```python
from build123d import *

# Parameters (mm, degrees)
CONG_1_R       = 1.1
ECHELLE1_SCALE = 0.69


with BuildPart() as part:
    # Esquisse1 → Révolution1 (revolve)
    with BuildSketch(Plane(origin=(0, 0, 0), x_dir=(0, 0, -1), z_dir=(1, 0, 0)), mode=Mode.PRIVATE) as r_volution1_sk:
        with BuildLine():
            Line((-7.5, 26), (-7.5, 21.2))
            Line((-7.5, 21.2), (-3.577708764, 21.2))
            ThreePointArc((-3.577708764, 21.2), (0, 22.8), (3.577708764, 21.2))
            Line((3.577708764, 21.2), (7.5, 21.2))
            Line((7.5, 21.2), (7.5, 26))
            Line((7.5, 26), (-7.5, 26))
        make_face()
    revolve(r_volution1_sk.sketch.rotate(Axis((0, 0, 0), (0, 0, -1)), 90), axis=Axis((0, 0, 0), (0, 0, -1)))

    # Congé1
    cong_1_edges = [part.edges().sort_by_distance(p)[0] for p in [
        (-26, 0, 7.5),
        (-26, 0, -7.5),
    ]]
    fillet(cong_1_edges, radius=CONG_1_R)


with BuildPart() as part_1:
    # Echelle1: scaled about (0, 0, 0)
    add(part.part.scale(ECHELLE1_SCALE))


solid = part_1.part
```
Could you check a few things on this model? Use its own coordinates, in mm. Coordinates: 2 decimals unless noted, no trailing zeros. Loops run counter-clockwise (first coordinate to the right, second up) from the corner with the lowest first, then second, coordinate; pieces in that order, holes last.
1) Imagine slicing it at A-A (x = 0). List the corners of the cut face in (y, z) for me (3 decimals).
Reported:
outline: (-17.94, -4.416) arc R0.759 ccw to (-17.181, -5.175) - (-14.628, -5.175) - (-14.628, -2.469) arc R3.312 cw to (-14.628, 2.469) - (-14.628, 5.175) - (-17.181, 5.175) arc R0.759 ccw to (-17.94, 4.416) - close; (14.628, -5.175) - (17.181, -5.175) arc R0.759 ccw to (17.94, -4.416) - (17.94, 4.416) arc R0.759 ccw to (17.181, 5.175) - (14.628, 5.175) - (14.628, 2.469) arc R3.312 cw to (14.628, -2.469) - close
2) Imagine slicing it at C-C (z = -3.5). List the corners of the cut face in (x, y) for me, and give its area (3 significant figures).
Reported:
outline: circle Ø35.88 at (0, 0); hole circle Ø29.26 at (0, 0)
area: 339 mm2
3) Will these pins go through, and if not, where does the flat tip stop? pin 1 Ø2 at (x, z) = (2.5, -0.5) entering from -Y; pin 2 Ø1 at (y, z) = (-5, -3.5) entering from -X; pin 3 Ø1.5 at (x, z) = (8.5, 0) entering from +Y.
Reported:
pin 1: stops at y = -17.88
pin 2: stops at x = -17.37
pin 3: stops at y = 16.18
4) Please list where these lines run through material, in increasing order: line 1 along Y through (x, z) = (0, -3.4); line 2 along Y through (x, z) = (-9, 2.5); line 3 along X through (y, z) = (-7, 2.25).
Reported:
line 1: y = -17.94 to -14.63, 14.63 to 17.94
line 2: y = -15.52 to -11.53, 11.53 to 15.52
line 3: x = -16.52 to -13.1, 13.1 to 16.52
5) Thinking about a two-plate mould opening in Y: for faces 1 (the face through (-3.17, 14.28, -3.84)), 2 (the face through (-3.17, 14.28, 3.8)), 3 (the face through (17.11, -5.39, 0.06)), 4 (the face through (-13, -8, -5.175)), which applies, released by +Y, released by -Y, zero draft, split by the parting line, or undercut?
Reported:
face 1: undercut
face 2: undercut
face 3: split by the parting line
face 4: zero draft
